from build123d import *

# Parameters (mm, degrees)
F0_R     = 57.15
F1_DEPTH = 12.7
F2_R     = 2.5527
F3_DEPTH = 12.7
F5_COUNT = 12
F6_R     = 2.5527
F7_DEPTH = 12.7
F8_COUNT = 12


with BuildPart() as f1:
    # F0 (on Top) → F1 (new body)
    with BuildSketch(Plane.XY):
        Circle(F0_R)
    extrude(amount=F1_DEPTH)

    # F2 (on face) → F3 (cut, through all)
    with BuildSketch(Plane.XY.offset(12.7)):
        with Locations((-52.3875, 0)):
            Circle(F2_R)
    f3 = extrude(amount=-F3_DEPTH, mode=Mode.SUBTRACT)

    # F5: F3 ×12 about axis
    f5_axis = Axis((0, 0, 5.419571884), (0, 0, -1))
    for i in range(1, F5_COUNT):
        add(f3.rotate(f5_axis, i * 360 / F5_COUNT), mode=Mode.SUBTRACT)

    # F6 (on face) → F7 (cut, through all)
    with BuildSketch(Plane.XY.offset(12.7)):
        with Locations((0, 38.1)):
            Circle(F6_R)
    f7 = extrude(amount=-F7_DEPTH, mode=Mode.SUBTRACT)

    # F8: F7 ×12 about axis
    f8_axis = Axis((0, 0, 5.419571884), (0, 0, -1))
    for i in range(1, F8_COUNT):
        add(f7.rotate(f8_axis, i * 360 / F8_COUNT), mode=Mode.SUBTRACT)


solid = f1.part
The model under review builds one solid part; all positions refer to its coordinate system, in mm. Round coordinates to 2 decimals unless told otherwise and drop trailing zeros. Write each loop counter-clockwise with the first axis right and the second up, starting at its lowest first coordinate (ties: lowest second). Pieces come first, ordered by that corner, then holes. Notation, with made-up numbers: M 41.25,4.25 L 91.25,4.25 A23 cw 91.25,35.25 Z; hole C 46.5,-35 d10. An arc over 180 degrees is marked long. Use a Markdown table: item, result. Add a question column.
Q1. To check wall thickness, follow line 1 (Y direction, x = 32.5, z = 1.5); line 2 (X direction, y = -46, z = 11.25); line 3 (Y direction, x = 45, z = 7.75). State the ranges of each line that lie inside material, in increasing order.
Q2. We need section C-C, the plane x = 19.05. State the section outline as (y, z) points, plus the area to 3 significant figures.
Q3. Insertion check: pin 1 (1.5 mm diameter, centred on y = 23, z = 8.5, fed in from +X); pin 2 (4 mm diameter, centred on x = -21, z = 2, fed in from +Y); pin 3 (6 mm diameter, centred on y = 37.5, z = 8, fed in from +X). Each pin has a flat end and moves straight along its axis. Give the tip position at first contact, or say it passes through.
Q4. We need section A-A, the plane y = 0. State the section outline as (x, z) points.
Q5. We need section D-D, the plane z = 3.75. Count the separate pieces of the cut face and the enclosed holes in it, plus the area to 3 significant figures.
Q6. The part is to be moulded in two halves that separate along X. For faces 1 (the face through (-1, 1, 12.7)), 2 (the face through (0.553, -35.608, 6.439)), 3 (the face through (-57.095, 2.513, 6.261)), say which applies: pulls with the +X half, pulls with the -X half, needs draft (parallel to the pull), parting line crosses it, or undercut.
Findings below:
| question | item | result |
|---|---|---|
| 1 | line 1 | y = -47.01 to -21.55, -16.55 to 16.55, 21.55 to 47.01 |
| 1 | line 2 | x = -33.91 to -28.67, -23.72 to 23.72, 28.67 to 33.91 |
| 1 | line 3 | y = -35.23 to -28.72, -23.67 to 23.67, 28.72 to 35.23 |
| 2 | outline | M -53.88,0 L -35.55,0 L -35.55,12.7 L -53.88,12.7 Z; M -30.44,0 L 30.44,0 L 30.44,12.7 L -30.44,12.7 Z; M 35.55,0 L 53.88,0 L 53.88,12.7 L 35.55,12.7 Z |
| 2 | area | 1,240 mm² |
| 3 | pin 1 | stops at x = 52.64 |
| 3 | pin 2 | stops at y = 53.9 |
| 3 | pin 3 | stops at x = 45.56 |
| 4 | outline | M -57.15,0 L -54.94,0 L -54.94,12.7 L -57.15,12.7 Z; M -49.83,0 L -40.65,0 L -40.65,12.7 L -49.83,12.7 Z; M -35.55,0 L 35.55,0 L 35.55,12.7 L -35.55,12.7 Z; M 40.65,0 L 49.83,0 L 49.83,12.7 L 40.65,12.7 Z; M 54.94,0 L 57.15,0 L 57.15,12.7 L 54.94,12.7 Z |
| 5 | separate pieces | 1 |
| 5 | enclosed holes | 24 |
| 5 | area | 9,770 mm² |
| 6 | face 1 | needs draft |
| 6 | face 2 | undercut |
| 6 | face 3 | parting line crosses it |
